The listing builds one solid part. Answer for the finished solid, in the listing's coordinates (mm). A direction names the side the tool comes from. Coordinates: 2 decimals unless noted, no trailing zeros. Order: outer loops, then holes, each group sorted by start corner. A loop starts at its lowest first (then second) coordinate and runs counter-clockwise, first axis right, second up. Notation, with made-up numbers: (73.5, 79.5) -> (86.5, 79.5) arc R25 ccw to (86.5, 118.5) -> close; hole circle Ø10 at (72.5, 41.25). An arc over 180 degrees is marked (long way). Answer in a Markdown table with one row per item. Add a question column.
```python
from build123d import *

# Parameters (mm, degrees)
SKETCH1_W           = 558.8
SKETCH1_H           = 342.9
SKETCH1_W_2         = 530.225
SKETCH1_H_2         = 298.45
BOSS_EXTRUDE1_DEPTH = 25.4
SKETCH2_W           = 530.225
SKETCH2_H           = 298.45
BOSS_EXTRUDE2_DEPTH = 2
SKETCH3_W           = 100
SKETCH3_H           = 100
BOSS_EXTRUDE3_DEPTH = 76.2


with BuildPart() as part:
    # Sketch1 → Boss-Extrude1 (new body)
    with BuildSketch(Plane.XY):
        Rectangle(SKETCH1_W, SKETCH1_H)
        with Locations((0, 7.9375)):
            Rectangle(SKETCH1_W_2, SKETCH1_H_2, mode=Mode.SUBTRACT)
    extrude(amount=-BOSS_EXTRUDE1_DEPTH)

    # Sketch2 → Boss-Extrude2 (add)
    with BuildSketch(Plane(origin=(0, 0, -25.4), x_dir=(-1, 0, 0), z_dir=(0, 0, -1))):
        with Locations((0, 7.9375)):
            Rectangle(SKETCH2_W, SKETCH2_H)
    extrude(amount=-BOSS_EXTRUDE2_DEPTH)

    # Sketch3 → Boss-Extrude3 (add)
    with BuildSketch(Plane(origin=(0, 0, -25.4), x_dir=(-1, 0, 0), z_dir=(0, 0, -1))):
        Rectangle(SKETCH3_W, SKETCH3_H)
    extrude(amount=BOSS_EXTRUDE3_DEPTH)


solid = part.part
```
Q1. Determine the mould class of faces 1 (the face through (-4, -141.288, -12)), 2 (the face through (66, 2, -25.4)), 3 (the face through (1, -50, -63)) for opening direction Y: +Y half, -Y half, draft (parallel to the pull), parting line (faces both ways), or undercut.
Q2. A cutting plane is placed at A-A (x = 196). Determine the outline of the cut face in (y, z), then the cut area to 3 significant figures.
Q3. Given pin 1 (23 mm diameter, centred on y = 13, z = -51.5, fed in from +X); pin 2 (3 mm diameter, centred on x = -196.5, y = 93.5, fed in from -Z); pin 3 (1 mm diameter, centred on x = -160, y = 108, fed in from +Z), each flat-ended and moving along its own axis, determine where each tip first touches the part or whether it passes through.
Q4. A cutting plane is placed at C-C (z = -38). Determine the outline of the cut face in (x, y).
Q5. Straight lines are drawn through the part: line 1 (Y direction, x = -18, z = -16); line 2 (X direction, y = 65, z = -14); line 3 (Z direction, x = 22.5, y = 154). For each, find the intervals that lie inside material, in ascending order.
Q6. For faces 4 (the face through (1, 50, -63)), 5 (the face through (265.112, 6, -12)), 6 (the face through (-50, -1, -63)), determine the directions among +Z, -Z, +X, -X, +Y, -Y from which every point of the face is accessible in a straight line to the end or side of a thin tool.
Q7. A cutting plane is placed at D-D (x = 40.5). Determine the outline of the cut face in (y, z).
Q8. A cutting plane is placed at B-B (y = 17). Determine the outline of the cut face in (x, z), then the cut area to 3 significant figures.
Returned:
| question | item | result |
|---|---|---|
| 1 | face 1 | undercut |
| 1 | face 2 | draft |
| 1 | face 3 | -Y half |
| 2 | outline | (-171.45, -25.4) -> (171.45, -25.4) -> (171.45, 0) -> (157.16, 0) -> (157.16, -23.4) -> (-141.29, -23.4) -> (-141.29, 0) -> (-171.45, 0) -> close |
| 2 | area | 1,730 mm² |
| 3 | pin 1 | stops at x = 50 |
| 3 | pin 2 | stops at z = -25.4 |
| 3 | pin 3 | stops at z = -23.4 |
| 4 | outline | (-50, -50) -> (50, -50) -> (50, 50) -> (-50, 50) -> close |
| 5 | line 1 | y = -171.45 to -141.29, 157.16 to 171.45 |
| 5 | line 2 | x = -279.4 to -265.11, 265.11 to 279.4 |
| 5 | line 3 | z = -25.4 to -23.4 |
| 6 | face 4 | -Z, +X, -X, +Y |
| 6 | face 5 | +Z |
| 6 | face 6 | -Z, -X, +Y, -Y |
| 7 | outline | (-171.45, -25.4) -> (-50, -25.4) -> (-50, -101.6) -> (50, -101.6) -> (50, -25.4) -> (171.45, -25.4) -> (171.45, 0) -> (157.16, 0) -> (157.16, -23.4) -> (-141.29, -23.4) -> (-141.29, 0) -> (-171.45, 0) -> close |
| 8 | outline | (-279.4, -25.4) -> (-50, -25.4) -> (-50, -101.6) -> (50, -101.6) -> (50, -25.4) -> (279.4, -25.4) -> (279.4, 0) -> (265.11, 0) -> (265.11, -23.4) -> (-265.11, -23.4) -> (-265.11, 0) -> (-279.4, 0) -> close |
| 8 | area | 9,410 mm² |
